Here's how the part is built. I have some questions about the finished solid (model axes, mm). Give positions to 0.01 mm unless a question says otherwise; leave off trailing zeros. Loops run counter-clockwise (first coordinate to the right, second up) from the corner with the lowest first, then second, coordinate; pieces in that order, holes last.
Q1. If we section it at D-D (y = 55.5): Please give me the cut outline in (x, z).
Q2. If we section it at C-C (x = 135): Please give me the cut outline in (y, z), plus the area to 3 significant figures.
Q3. I need wall thicknesses on line 1 (Y direction, x = 180, z = 2.5); line 2 (Y direction, x = 53, z = 6.5); line 3 (Y direction, x = 158, z = 6). Which ranges of each line are inside material? Lowest first, please.
Q4. If we section it at B-B (y = 69.5): Please give me the cut outline in (x, z), plus the area to 3 significant figures.
Q5. If we section it at A-A (x = 39): Please give me the cut outline in (y, z).
Q6. Will this pin go through, and if not, where does the flat tip stop? P1, Ø1.5, axis at x = 50.5, y = 33.5, coming from the -Z side.
from build123d import *

# Parameters (mm, degrees)
SKETCH1_W           = 248.984951577
SKETCH1_H           = 120.432938534
SKETCH1_R           = 3.927622284
BOSS_EXTRUDE1_DEPTH = 10


with BuildPart() as part:
    # Sketch1 → Boss-Extrude1 (new body)
    with BuildSketch(Plane.XY):
        with Locations((115.469095844, 55.276599595)):
            Rectangle(SKETCH1_W, SKETCH1_H)
        with BuildLine():
            Line((0, 32.653955718), (15.621240173, 32.653955718))
            ThreePointArc((15.621240173, 32.653955718), (30.388379433, 16.62799554), (15.621240173, 0.602035363))
            Line((15.621240173, 0.602035363), (10.293959075, 0.602035363))
            Line((10.293959075, 0.602035363), (10.293959075, 8.861852454))
            Line((10.293959075, 8.861852454), (14.274680474, 8.861852454))
            ThreePointArc((14.274680474, 8.861852454), (22.080061465, 16.061509913), (15.621240173, 24.490191155))
            Line((15.621240173, 24.490191155), (8.429804398, 24.490191155))
            Line((8.429804398, 24.490191155), (8.429804398, 0.602035363))
            Line((8.429804398, 0.602035363), (0, 0.602035363))
            Line((0, 0.602035363), (0, 32.653955718))
        make_face(mode=Mode.SUBTRACT)
        with BuildLine():
            Line((53.313679211, 11.346247394), (53.313679211, 18.830088837))
            Line((53.313679211, 18.830088837), (69.812648012, 18.830088837))
            ThreePointArc((69.812648012, 18.830088837), (38.193038875, 9.668726743), (65.717255622, 27.728287366))
            Line((65.717255622, 27.728287366), (59.75927661, 22.396332813))
            ThreePointArc((59.75927661, 22.396332813), (44.669643003, 16.311643284), (60.163684849, 11.346247394))
            Line((60.163684849, 11.346247394), (53.313679211, 11.346247394))
        make_face(mode=Mode.SUBTRACT)
        Polygon((83.185651108, 0.602035363), (74.742166319, 0.602035363), (86.191958884, 32.653955718), (94.215171192, 32.653955718), (105.915689142, 0.602035363), (97.223875808, 0.602035363), (90.044966021, 20.267647237), (87.696137012, 14.219111042), (90.567743799, 14.219111042), (93.405960474, 6.444216356), (85.272632474, 6.444216356), align=None, mode=Mode.SUBTRACT)
        Polygon((165.929478775, 74.975053885), (141.623819181, 91.5963268), (218.812994732, 91.5963268), (195.166908856, 73.782247188), (188.229793622, 73.782247188), (188.229793622, 65.193610278), (196.812613934, 65.193610278), (196.812613934, 72.134215516), (220.35325448, 89.868856548), (220.35325448, 39.050837541), (204.652216255, 45.070871149), (220.35325448, 34.108892188), (220.35325448, 1.27565402), (218.022003488, 1.27565402), (200.124503338, 28.805885142), (211.866175411, 1.27565402), (168.723408334, 1.27565402), (179.195250301, 39.239610221), (160.65924824, 1.27565402), (137.714117569, 1.27565402), (165.322421142, 35.525080037), (130.296961385, 1.27565402), (126.146157188, 1.27565402), (126.146157188, 20.267647237), (165.929478775, 49.461736063), (126.146157188, 25.486362594), (126.146157188, 91.54755974), (132.709440168, 91.54755974), align=None, mode=Mode.SUBTRACT)
        with BuildLine():
            Line((4.834579987, 57.798227986), (0, 64.897937367))
            ThreePointArc((0, 64.897937367), (50.085795072, 86.302645706), (103.604066377, 96.428999618))
            ThreePointArc((103.604066377, 96.428999618), (52.480961252, 81.558182411), (4.834579987, 57.798227986))
        make_face(mode=Mode.SUBTRACT)
        Polygon((35.321567329, 31.069910316), (44.509426528, 61.76571264), (48.564924823, 63.753147229), (42.461506674, 43.362182051), (88.328778824, 90.179245039), (96.659761905, 93.678257933), align=None, mode=Mode.SUBTRACT)
        with Locations((76.813345198, 105.179515455)):
            Circle(SKETCH1_R, mode=Mode.SUBTRACT)
    extrude(amount=BOSS_EXTRUDE1_DEPTH)


solid = part.part
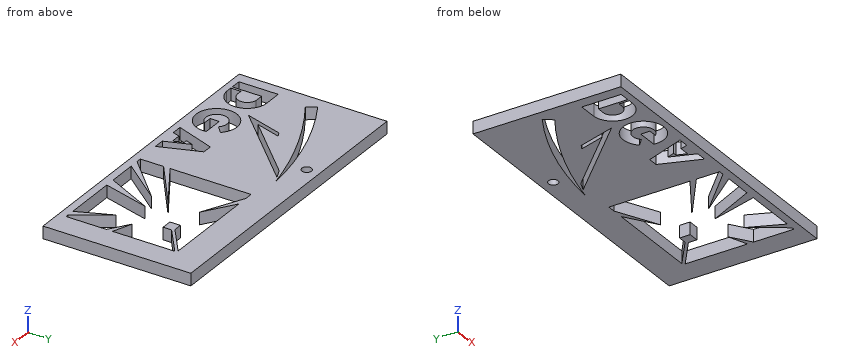
Check sheet entries:
1. outline: (-9.02, 0) - (42.63, 0) - (42.63, 10) - (-9.02, 10) - close; (46.09, 0) - (54.35, 0) - (54.35, 10) - (46.09, 10) - close; (59.26, 0) - (126.15, 0) - (126.15, 10) - (59.26, 10) - close; (220.35, 0) - (239.96, 0) - (239.96, 10) - (220.35, 10) - close
2. outline: (-4.94, 0) - (5.87, 0) - (5.87, 10) - (-4.94, 10) - close; (26.76, 0) - (30.82, 0) - (30.82, 10) - (26.76, 10) - close; (90.4, 0) - (115.49, 0) - (115.49, 10) - (90.4, 10) - close
2. area: 400 mm2
3. line 1: y = -4.94 to 1.28, 91.6 to 115.49
3. line 2: y = -4.94 to -0.01, 7.98 to 25.27, 33.27 to 49.11, 54.12 to 81.76, 87.17 to 115.49
3. line 3: y = -4.94 to 1.28, 26.44 to 28.36, 43.64 to 44.68, 78.93 to 80.4, 91.6 to 115.49
4. outline: (-9.02, 0) - (8.57, 0) - (8.57, 10) - (-9.02, 10) - close; (25.65, 0) - (68.07, 0) - (68.07, 10) - (25.65, 10) - close; (72.97, 0) - (126.15, 0) - (126.15, 10) - (72.97, 10) - close; (188.23, 0) - (196.81, 0) - (196.81, 10) - (188.23, 10) - close; (220.35, 0) - (239.96, 0) - (239.96, 10) - (220.35, 10) - close
4. area: 1,410 mm2
5. outline: (-4.94, 0) - (8.13, 0) - (8.13, 10) - (-4.94, 10) - close; (25.12, 0) - (34.82, 0) - (34.82, 10) - (25.12, 10) - close; (43.36, 0) - (75.9, 0) - (75.9, 10) - (43.36, 10) - close; (82.65, 0) - (115.49, 0) - (115.49, 10) - (82.65, 10) - close
6. P1: stops at z = 0
